Here's how the part is built. I have some questions about the finished solid (model axes, mm). Coordinates: 2 decimals unless noted, no trailing zeros. Loops run counter-clockwise (first coordinate to the right, second up) from the corner with the lowest first, then second, coordinate; pieces in that order, holes last. Notation, with made-up numbers: (63.5, -11) -> (89.5, -11) arc R19 ccw to (89.5, 22) -> close; hole circle Ø11 at (26, 29). An arc over 180 degrees is marked (long way). Answer as a JSON object with one key per item and string values. Group by question number.
1) I'm going to push flat-ended pins straight in: pin 1 (4 mm diameter, centred on x = 5, z = 2.5, fed in from -Y); pin 2 (1 mm diameter, centred on y = 7, z = 8.5, fed in from +X); pin 3 (5 mm diameter, centred on y = 6, z = 6, fed in from +X). Where does each tip first touch, or does it pass through?
2) If we mould it in two halves opening along Y, with no side actions, what happens to faces 1 (the cylindrical face through (2.29, 6.09, 3.88)), 2 (the flat face through (3, 12, 6)), 3 (the flat face through (3, 9, 0))? For each: +Y half, -Y half, draft (parallel to the pull), parting line (faces both ways), or undercut.
3) I need wall thicknesses on probe 1 along Z at (x, y) = (4.7, 6); probe 2 along X at (y, z) = (8.5, 6); probe 3 along Z at (x, y) = (3.5, 5.25). Which ranges of each line are inside material? Lowest first, please. Write a range as [from, to].
4) I want a section at A-A (z = 6). Write out the boundary of the cut face in (x, y).
5) I want a section at D-D (x = 7.75). Write out the boundary of the cut face in (y, z).
6) I want a section at C-C (y = 10). Write out the boundary of the cut face in (x, z).
7) I want a section at B-B (x = 1.25). Write out the boundary of the cut face in (y, z), then the cut area to 3 significant figures.
```python
from build123d import *

# Parameters (mm, degrees)
BOSS_EXTRU_1_DEPTH      = 12
ESQUISSE2_R             = 2.12
ENL_V_MAT_EXTRU_1_DEPTH = 12
ESQUISSE3_R             = 2.12
ENL_V_MAT_EXTRU_2_DEPTH = 12


with BuildPart() as part:
    # Esquisse1 → Boss.-Extru.1 (new body)
    with BuildSketch(Plane.XY):
        Polygon((0, 0), (0, 12), (12, 12), align=None)
    extrude(amount=BOSS_EXTRU_1_DEPTH)

    # Esquisse2 → Enlèv. mat.-Extru.1 (cut)
    with BuildSketch(Plane(origin=(0, 12, 0), x_dir=(1, 0, 0), z_dir=(0, 1, 0))):
        with Locations(Location((6, -6, 0), (0, 0, 270))):
            Circle(ESQUISSE2_R)
    extrude(amount=-ENL_V_MAT_EXTRU_1_DEPTH, mode=Mode.SUBTRACT)

    # Esquisse3 → Enlèv. mat.-Extru.2 (cut)
    with BuildSketch(Plane.ZY):
        with Locations((6, 6)):
            Circle(ESQUISSE3_R)
    extrude(amount=-ENL_V_MAT_EXTRU_2_DEPTH, mode=Mode.SUBTRACT)


solid = part.part
```
Determined:
{
 "1": {"pin 1": "y = 3", "pin 2": "x = 7.5", "pin 3": "x = 8.5"},
 "2": {"face 1": "undercut", "face 2": "+Y half", "face 3": "draft"},
 "3": {"probe 1": "[0, 3.88], [8.12, 12]", "probe 2": "[0, 3.88], [8.12, 8.5]", "probe 3": "[0, 4.02], [7.98, 12]"},
 "4": {"outline": "(0, 0) -> (3.88, 3.88) -> (0, 3.88) -> close; (0, 8.12) -> (3.88, 8.12) -> (3.88, 12) -> (0, 12) -> close; (8.12, 8.12) -> (12, 12) -> (8.12, 12) -> close"},
 "5": {"outline": "(7.75, 0) -> (12, 0) -> (12, 4.8) -> (7.75, 4.8) -> close; (7.75, 7.2) -> (12, 7.2) -> (12, 12) -> (7.75, 12) -> close"},
 "6": {"outline": "(0, 0) -> (10, 0) -> (10, 12) -> (0, 12) -> close; hole circle Ø4.24 at (6, 6)"},
 "7": {"outline": "(1.25, 0) -> (12, 0) -> (12, 12) -> (1.25, 12) -> close; hole circle Ø4.24 at (6, 6)", "area": "115 mm^2"}
}
